Autodesk Inventor part; units mm, degrees
ref_plane "YZ Plane" through (0, 0, 0) normal (1, 0, 0) x (0, 1, 0)
ref_plane "XZ Plane" through (0, 0, 0) normal (0, 1, 0) x (-1, 0, 0)
ref_plane "XY Plane" through (0, 0, 0) normal (0, 0, 1) x (1, 0, 0)
sketch "スケッチ1" plane through (0, 0, 0) normal (0, 0, 1) x (1, 0, 0)
  circle A0 centre (0, 0) radius 2
  dimension "d0" = 4
extrude "押し出し1" add sketch "スケッチ1" along normal blind 6
sketch "スケッチ2" plane through (0, 0, 6) normal (0, 0, 1) x (1, 0, 0)
  circle A0 centre (0, 0) radius 2
  circle A1 centre (0, 0) radius 4
  dimension "d3" = 8
extrude "押し出し2" add sketch "スケッチ2" along normal blind 2.6 contours A0 | A1
fillet "フィレット1" radius 2.6 1 edges at (-4, 0, 8.6)
thread "ねじ1"
sketch "スケッチ3" plane through (0, 0, 0) normal (0, 0, -1) x (-1, 0, 0)
  circle A0 centre (0, 0) radius 2
extrude "押し出し3" add sketch "スケッチ3" along normal blind 9
properties part number "SB　m4 15mmなべネジ" material "Steel, Mild"
For this review, take the finished solid that the model builds, in its own axes (mm). A direction names the side the tool comes from. Give positions to 0.01 mm unless a question says otherwise; leave off trailing zeros. Order: outer loops, then holes, each group sorted by start corner. A loop starts at its lowest first (then second) coordinate and runs counter-clockwise, first axis right, second up.
1) Wall thickness on line 1 (X direction, y = 3, z = 6.75); line 2 (Y direction, x = -1.5, z = 4.25); line 3 (X direction, y = 1.75, z = -1): over which ranges is each line inside the solid? List them lowest first.
2) Insertion check: pin 1 (1.5 mm diameter, centred on x = 0, z = -4, fed in from -Y); pin 2 (1 mm diameter, centred on x = -0.5, z = 0, fed in from +Y); pin 3 (2 mm diameter, centred on x = -2.5, y = 1.5, fed in from -Z); pin 4 (1 mm diameter, centred on x = 1, z = 0.5, fed in from -Y). Each pin has a flat end and moves straight along its axis. Give the tip position at first contact, or say it passes through.
3) For faces 1 (the face through (0, 0, 8.6)), 2 (the face through (-2, -1, 6)), list the 3-axis set-ups (+Z, -Z, +X, -X, +Y, -Y) from which the entire face can be reached by the end or side of a thin tool; tool diameter is ignored.
4) Take a section at A-A (z = -1). Give the boundary of the cut face in (x, y).
Derived:
1. line 1: x = -2.48 to 2.48
1. line 2: y = -1.32 to 1.32
1. line 3: x = -0.97 to 0.97
2. pin 1: stops at y = -2
2. pin 2: stops at y = 2
2. pin 3: stops at z = -9
2. pin 4: stops at y = -1.94
3. face 1: +Z, +X, -X, +Y, -Y
3. face 2: -Z
4. outline: circle Ø4 at (0, 0)
